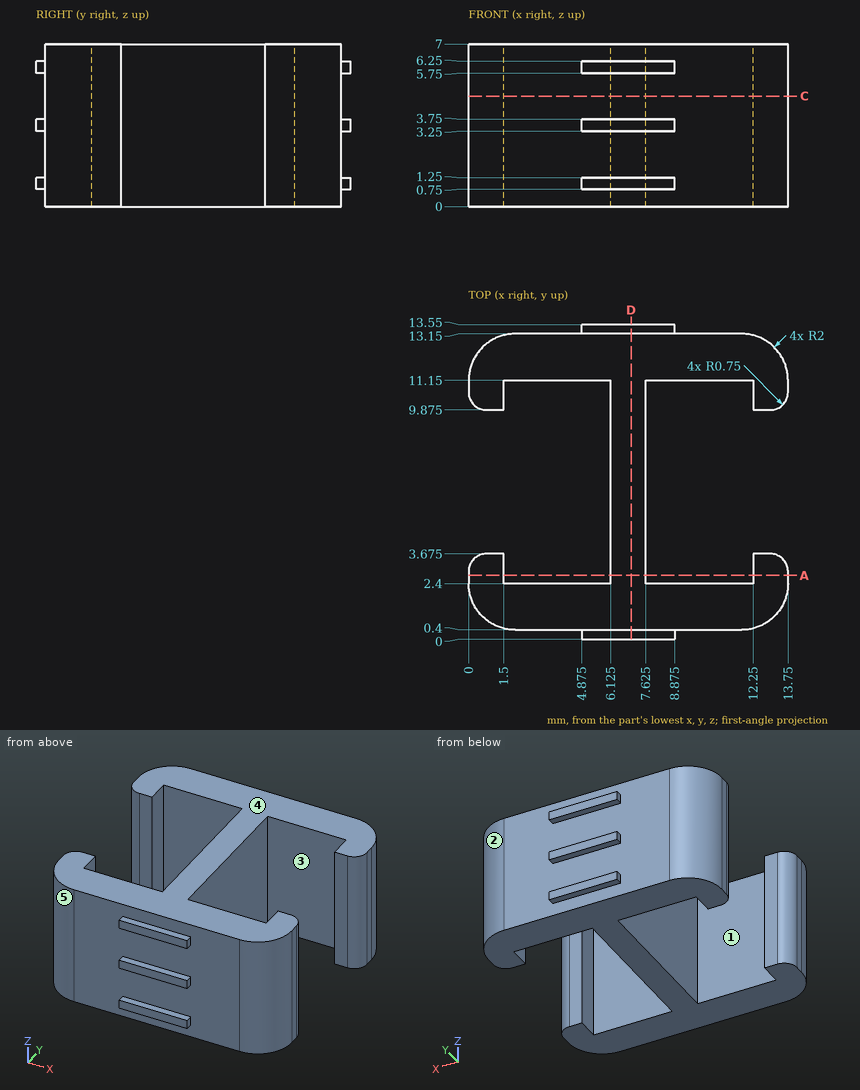
Verification items for this drawing (mm, ordinates from the low corner). A direction names the side the tool comes from. Coordinates: 2 decimals unless noted, no trailing zeros. Write each loop counter-clockwise with the first axis right and the second up, starting at its lowest first coordinate (ties: lowest second). Pieces come first, ordered by that corner, then holes. Notation, with made-up numbers: M -7.5,73 L 21.5,73 A35 cw 21.5,112 Z; hole C 57.5,72.25 d8. An arc over 180 degrees is marked long. Answer as a JSON object with one key per item and string values. Group by question number.
(1) Gauge pin test, flat ends, axial feed: pin 1 (1 mm diameter, centred on x = 2, z = 3.5, fed in from -Y); pin 2 (3 mm diameter, centred on x = 10.5, z = 4, fed in from +Y). Record the tip position at first contact, or that the pin passes through.
(2) Release check for a two-part mould opening along Y. For the marked faces 3, 4 and 5 record: +Y half, -Y half, draft (parallel to the pull), parting line (faces both ways), or undercut.
(3) Cross-section at A-A, the plane y = 2.75. Record the cut outline in (x, z) (3 decimals), and give its area (3 significant figures).
(4) Cross-section at D-D, the plane x = 7. Record the cut outline in (y, z), and give its area (4 significant figures).
(5) Cross-section at C-C, the plane z = 4.75. Record the cut outline in (x, y) (3 decimals).
(6) Tool access check on the marked faces 1 and 2. Record the directions out of +Z, -Z, +X, -X, +Y, -Y that give a thin tool (end or side, any length) a straight path to the whole face; none if there is none.
(7) Material ranges on line 1 (Y direction, x = 9.75, z = 5); line 2 (Y direction, x = 5, z = 6); line 3 (X direction, y = 4, z = 2.75) (3 decimals), recorded low to high.
Reply:
{
 "1": {"pin 1": "y = 0.4", "pin 2": "y = 13.15"},
 "2": {"face 3": "undercut", "face 4": "draft", "face 5": "-Y half"},
 "3": {"outline": "M 0,0 L 1.5,0 L 1.5,7 L 0,7 Z; M 6.125,0 L 7.625,0 L 7.625,7 L 6.125,7 Z; M 12.25,0 L 13.75,0 L 13.75,7 L 12.25,7 Z", "area": "31.5 mm²"},
 "4": {"outline": "M 0,0.75 L 0.4,0.75 L 0.4,0 L 13.15,0 L 13.15,0.75 L 13.55,0.75 L 13.55,1.25 L 13.15,1.25 L 13.15,3.25 L 13.55,3.25 L 13.55,3.75 L 13.15,3.75 L 13.15,5.75 L 13.55,5.75 L 13.55,6.25 L 13.15,6.25 L 13.15,7 L 0.4,7 L 0.4,6.25 L 0,6.25 L 0,5.75 L 0.4,5.75 L 0.4,3.75 L 0,3.75 L 0,3.25 L 0.4,3.25 L 0.4,1.25 L 0,1.25 Z", "area": "90.45 mm²"},
 "5": {"outline": "M 0,2.4 A2 ccw 2,0.4 L 11.75,0.4 A2 ccw 13.75,2.4 L 13.75,2.925 A0.75 ccw 13,3.675 L 12.25,3.675 L 12.25,2.4 L 7.625,2.4 L 7.625,11.15 L 12.25,11.15 L 12.25,9.875 L 13,9.875 A0.75 ccw 13.75,10.625 L 13.75,11.15 A2 ccw 11.75,13.15 L 2,13.15 A2 ccw 0,11.15 L 0,10.625 A0.75 ccw 0.75,9.875 L 1.5,9.875 L 1.5,11.15 L 6.125,11.15 L 6.125,2.4 L 1.5,2.4 L 1.5,3.675 L 0.75,3.675 A0.75 ccw 0,2.925 Z"},
 "6": {"face 1": "+Z, -Z", "face 2": "+Z, -Z, +X, +Y"},
 "7": {"line 1": "0.4 to 2.4, 11.15 to 13.15", "line 2": "0 to 2.4, 11.15 to 13.55", "line 3": "6.125 to 7.625"}
}
